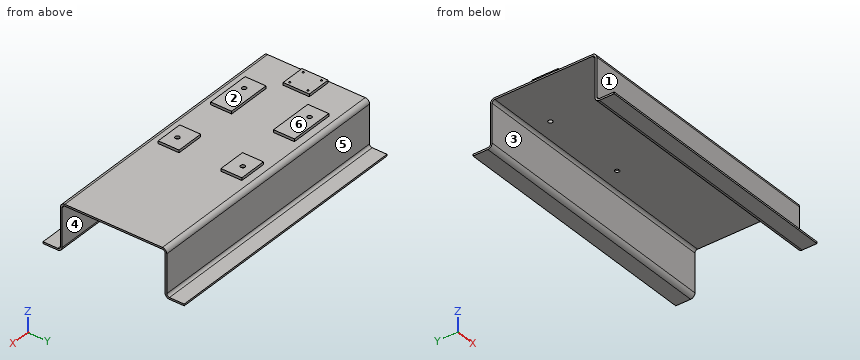
```python
from build123d import *

# Parameters (mm, degrees)
F0_W     = 1911.35
F0_H     = 774.7
F0_W_2   = 323.85
F0_H_2   = 152.4
F0_W_3   = 203.2
F0_R     = 15.875
F1_DEPTH = 12.7
F2_DEPTH = 19.05
F3_W     = 12.7
F3_H     = 330.2
F3_H_2   = 12.7
F3_W_2   = 127
F4_DEPTH = 1911.35
F5_R     = 19.05
F6_R     = 31.75
F7_R     = 7.14375
F8_DEPTH = 19.05


with BuildPart() as f1:
    # F0 (on Top) → F1 (new body)
    with BuildSketch(Plane.XY):
        Rectangle(F0_W, F0_H)
        with Locations((-516.128, -228.6)):
            Rectangle(F0_W_2, F0_H_2, mode=Mode.SUBTRACT)
        with Locations((39.497, -228.6)):
            Rectangle(F0_W_3, F0_H_2, mode=Mode.SUBTRACT)
        with Locations((-516.128, 228.6)):
            Rectangle(F0_W_2, F0_H_2, mode=Mode.SUBTRACT)
        with Locations((39.497, 228.6)):
            Rectangle(F0_W_3, F0_H_2, mode=Mode.SUBTRACT)
        with Locations((-516.128, 228.6)):
            Rectangle(F0_W_2, F0_H_2)
        with Locations((-582.803, 238.252)):
            Circle(F0_R, mode=Mode.SUBTRACT)
        with Locations((-516.128, -228.6)):
            Rectangle(F0_W_2, F0_H_2)
        with Locations((-582.803, -238.252)):
            Circle(F0_R, mode=Mode.SUBTRACT)
        with Locations((39.497, 228.6)):
            Rectangle(F0_W_3, F0_H_2)
        with Locations((45.847, 238.252)):
            Circle(F0_R, mode=Mode.SUBTRACT)
        with Locations((39.497, -228.6)):
            Rectangle(F0_W_3, F0_H_2)
        with Locations((45.847, -238.252)):
            Circle(F0_R, mode=Mode.SUBTRACT)
    extrude(amount=-F1_DEPTH)

    # F0 (on Top) → F2 (join)
    with BuildSketch(Plane.XY):
        with Locations((-516.128, 228.6)):
            Rectangle(F0_W_2, F0_H_2)
        with Locations((-582.803, 238.252)):
            Circle(F0_R, mode=Mode.SUBTRACT)
        with Locations((-516.128, -228.6)):
            Rectangle(F0_W_2, F0_H_2)
        with Locations((-582.803, -238.252)):
            Circle(F0_R, mode=Mode.SUBTRACT)
        with Locations((39.497, 228.6)):
            Rectangle(F0_W_3, F0_H_2)
        with Locations((45.847, 238.252)):
            Circle(F0_R, mode=Mode.SUBTRACT)
        with Locations((39.497, -228.6)):
            Rectangle(F0_W_3, F0_H_2)
        with Locations((45.847, -238.252)):
            Circle(F0_R, mode=Mode.SUBTRACT)
    extrude(amount=F2_DEPTH)

    # F3 (on face) → F4 (join)
    with BuildSketch(Plane.YZ.offset(955.675)):
        with Locations((-381, -165.1)):
            Rectangle(F3_W, F3_H)
        with Locations((-381, -336.55)):
            Rectangle(F3_W, F3_H_2)
        with Locations((-450.85, -336.55)):
            Rectangle(F3_W_2, F3_H_2)
        with Locations((381, -165.1)):
            Rectangle(F3_W, F3_H)
        with Locations((450.85, -336.55)):
            Rectangle(F3_W_2, F3_H_2)
        with Locations((381, -336.55)):
            Rectangle(F3_W, F3_H_2)
    extrude(amount=-F4_DEPTH)

    # F5
    f5_edges = [f1.edges().sort_by_distance(p)[0] for p in [
        (0, -387.35, -330.2),
        (0, 387.35, -330.2),
        (0, 374.65, -12.7),
        (0, -374.65, -12.7),
    ]]
    fillet(f5_edges, radius=F5_R)

    # F6
    f6_edges = [f1.edges().sort_by_distance(p)[0] for p in [
        (0, 374.65, -342.9),
        (0, -374.65, -342.9),
        (0, 387.35, 0),
        (0, -387.35, 0),
    ]]
    fillet(f6_edges, radius=F6_R)

    # F7 (on face) → F8 (join)
    with BuildSketch(Plane.XY):
        Polygon((-765.429, -95.25), (-765.429, 0), (-765.429, 95.25), (-943.229, 95.25), (-943.229, 0), (-943.229, -95.25), align=None)
        with Locations((-917.575, -66.548)):
            Circle(F7_R, mode=Mode.SUBTRACT)
        with Locations((-790.575, -66.548)):
            Circle(F7_R, mode=Mode.SUBTRACT)
        with Locations((-917.575, 66.548)):
            Circle(F7_R, mode=Mode.SUBTRACT)
        with Locations((-790.575, 66.548)):
            Circle(F7_R, mode=Mode.SUBTRACT)
    extrude(amount=F8_DEPTH)


solid = f1.part
```
Read the model definition and answer for the solid it produces. Units are mm, in the model's axes. Face numbers are marked on the shaded views. A direction names the side the tool comes from. Give positions to 0.01 mm unless a question says otherwise; leave off trailing zeros. Order: outer loops, then holes, each group sorted by start corner. A loop starts at its lowest first (then second) coordinate and runs counter-clockwise, first axis right, second up. Notation, with made-up numbers: (39.5, 57) -> (49.5, 57) arc R27 ccw to (49.5, 88) -> close; hole circle Ø6 at (32.25, 48). An arc over 180 degrees is marked (long way). One line per item, written item: value. Start each with the question number.
(1) The part is cut by section B-B (x = 818.5). Determine the outline of the cut face in (y, z), and give its area (3 significant figures).
(2) A tool of negligible diameter and unlimited length cuts with its end or side. For the marked faces 4, 5 and 6, from which of +Z, -Z, +X, -X, +Y, -Y can it reach the whole face along a straight path? Write none if from no direction.
(3) Straight lines are drawn through the part: L1, parallel to Y at x = 191, z = -300.5; L2, parallel to Y at x = -359, z = 2.5; L3, parallel to Z at x = 645.5, y = 264. For each, find the intervals that lie inside material, in ascending order.
(4) Flat-ended cylindrical pins translate along their axes: P1, Ø1, axis at x = -444.5, z = -64.5, coming from the +Y side; P2, Ø8, axis at x = 661, y = -204, coming from the +Z side; P3, Ø5, axis at x = 67.5, z = -154.5, coming from the -Y side. Find the tip coordinate at first contact, or state that the pin passes through.
(5) For a pull along Y with two mould halves and no side action, classify the marked faces 1, 2 and 3 as released by +Y, released by -Y, zero draft, split by the parting line, or undercut.
(6) The part is cut by section C-C (y = -281). Determine the outline of the cut face in (x, z) (3 decimals).
(7) The part is cut by section A-A (z = -119). Determine the outline of the cut face in (x, y) (3 decimals).
(8) The part is cut by section D-D (y = -17.5). Determine the outline of the cut face in (x, z) (3 decimals).
Taken from the geometry:
1. outline: (-514.35, -342.9) -> (-406.4, -342.9) arc R31.75 ccw to (-374.65, -311.15) -> (-374.65, -31.75) arc R19.05 cw to (-355.6, -12.7) -> (355.6, -12.7) arc R19.05 cw to (374.65, -31.75) -> (374.65, -311.15) arc R31.75 ccw to (406.4, -342.9) -> (514.35, -342.9) -> (514.35, -330.2) -> (406.4, -330.2) arc R19.05 cw to (387.35, -311.15) -> (387.35, -31.75) arc R31.75 ccw to (355.6, 0) -> (-355.6, 0) arc R31.75 ccw to (-387.35, -31.75) -> (-387.35, -311.15) arc R19.05 cw to (-406.4, -330.2) -> (-514.35, -330.2) -> close
1. area: 20,900 mm^2
2. face 4: -Z, +X, -X
2. face 5: +Z, +X, -X, +Y
2. face 6: +Z, +X, -X, +Y, -Y
3. L1: -387.35 to -374.65, 374.65 to 387.35
3. L2: -304.8 to -152.4, 152.4 to 304.8
3. L3: -12.7 to 0
4. P1: y = 387.35
4. P2: z = 0
4. P3: y = -387.35
5. face 1: released by -Y
5. face 2: zero draft
5. face 3: undercut
6. outline: (-955.675, -12.7) -> (955.675, -12.7) -> (955.675, 0) -> (141.097, 0) -> (141.097, 19.05) -> (-62.103, 19.05) -> (-62.103, 0) -> (-354.203, 0) -> (-354.203, 19.05) -> (-678.053, 19.05) -> (-678.053, 0) -> (-955.675, 0) -> close
7. outline: (-955.675, -387.35) -> (955.675, -387.35) -> (955.675, -374.65) -> (-955.675, -374.65) -> close; (-955.675, 374.65) -> (955.675, 374.65) -> (955.675, 387.35) -> (-955.675, 387.35) -> close
8. outline: (-955.675, -12.7) -> (955.675, -12.7) -> (955.675, 0) -> (-765.429, 0) -> (-765.429, 19.05) -> (-943.229, 19.05) -> (-943.229, 0) -> (-955.675, 0) -> close
